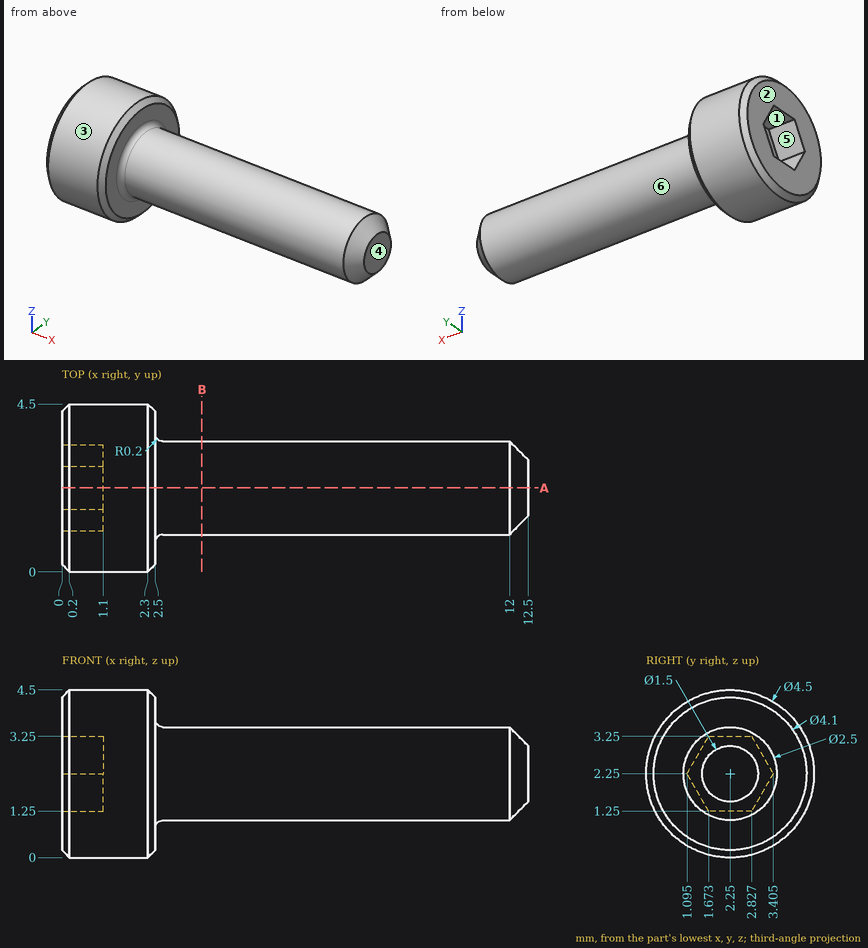
Input: dimensioned drawing with shaded views. Units: mm. Origin: part minimum x, y, z. A direction names the side the tool comes from. Give positions to 0.01 mm unless a question says otherwise; leave off trailing zeros. Loops run counter-clockwise (first coordinate to the right, second up) from the corner with the lowest first, then second, coordinate; pieces in that order, holes last. Notation, with made-up numbers: (6.25, 89) - (10.25, 89) arc R21 ccw to (10.25, 127) - close; hole circle Ø4 at (29, -36). An arc over 180 degrees is marked (long way). Answer as CSV lines item,"result". Start each with the question number.
(1) Ray query, line 1 along Y through (x, z) = (3.75, 3.25); line 2 along X through (y, z) = (2.75, 4.1); line 3 along Z through (x, y) = (3.25, 2.25). Return the intervals inside material, ascending. Write a range as [from, to].
(2) Pin query (flat end, axial travel): P1, Ø2, axis at x = 7.5, z = 1.5, coming from the +Y side; P2, Ø1, axis at x = 4.5, z = 2, coming from the -Y side; P3, Ø1.5, axis at x = 2.5, y = 3.5, coming from the +Z side. Return the tip coordinate at first contact, or that it passes through.
(3) Section query A-A (y = 2.25). Output: boundary loops of the cut face in (x, z).
(4) Mould query, pull axis Z, two halves, no side actions, for the marked faces 1, 2 and 3. Classes: +Z half, -Z half, draft (parallel to the pull), parting line (faces both ways), or undercut.
(5) Reachability of the marked faces 4, 5 and 6 from +Z, -Z, +X, -X, +Y, -Y: full face, straight path, thin tool, end or side. Return the list, or none.
(6) Section query B-B (x = 3.75). Output: boundary loops of the cut face in (y, z).
Worked answers:
1,line 1,"y = [1.5, 3]"
1,line 2,"x = [0, 2.5]"
1,line 3,"z = [1, 3.5]"
2,P1,"stops at y = 3.5"
2,P2,"stops at y = 1"
2,P3,"stops at z = 4.44"
3,outline,"(0, 0.2) - (0.2, 0) - (2.3, 0) - (2.5, 0.2) - (2.5, 0.8) arc R0.2 cw to (2.7, 1) - (12, 1) - (12.5, 1.5) - (12.5, 3) - (12, 3.5) - (2.7, 3.5) arc R0.2 cw to (2.5, 3.7) - (2.5, 4.3) - (2.3, 4.5) - (0.2, 4.5) - (0, 4.3) - (0, 3.25) - (1.1, 3.25) - (1.1, 1.25) - (0, 1.25) - close"
4,face 1,"undercut"
4,face 2,"draft"
4,face 3,"parting line"
5,face 4,"+Z, -Z, +X, +Y, -Y"
5,face 5,"-X"
5,face 6,"+X"
6,outline,"circle Ø2.5 at (2.25, 2.25)"
